Design review of the part built by this model. Coordinates are the model's own, in mm. A direction names the side the tool comes from. Give positions to 0.01 mm unless a question says otherwise; leave off trailing zeros. Write each loop counter-clockwise with the first axis right and the second up, starting at its lowest first coordinate (ties: lowest second). Pieces come first, ordered by that corner, then holes. Notation, with made-up numbers: M 68.25,-10 L 83.25,-10 A19 ccw 83.25,16 Z; hole C -34,37.25 d8. An arc over 180 degrees is marked long. Use a Markdown table: item, result. Add a question column.
Autodesk Inventor part; units mm, degrees
ref_plane "YZ Plane" through (0, 0, 0) normal (1, 0, 0) x (0, 1, 0)
ref_plane "XZ Plane" through (0, 0, 0) normal (0, 1, 0) x (-1, 0, 0)
ref_plane "XY Plane" through (0, 0, 0) normal (0, 0, 1) x (1, 0, 0)
sketch "Sketch1" plane through (0, 0, 0) normal (0, 0, 1) x (1, 0, 0)
  line L0 (-250, -250) -> (250, -250)
  line L1 (250, -250) -> (250, 250)
  line L2 (250, 250) -> (-250, 250)
  line L3 (-250, 250) -> (-250, -250)
  line L4 (-250, -250) -> (250, 250) construction
  line L5 (250, -250) -> (-250, 250) construction
  point P0 (0, 0)
  dimension "d0" = 500
  dimension "d1" = 500
extrude "Extrusion1" add sketch "Sketch1" along normal blind 300
shell "Shell1" thickness 10 removed faces 2 at (83.3333, -83.3333, 0) at (83.3333, -83.3333, 300)
sketch "Sketch2" plane through (0, 0, 0) normal (1, 0, 0) x (0, 1, 0)
  line L0 (-250, 0) -> (250, 0) construction
  line L1 (250, 0) -> (250, 300) construction
  line L2 (-250, 300) -> (250, 300) construction
  line L3 (-250, 0) -> (-250, 300) construction
  line L4 (-250, 0) -> (-250, 300) construction
  line L5 (-250, 150) -> (250, 150) construction
  circle A0 centre (0, 150) radius 30
  arc A1 (205, 115) -> (17.4379, 125.5885) centre (104.6273, 3.5311) ccw
  arc A2 (160.6867, 200) -> (-12.382, 177.3256) centre (111.438, -95.93) ccw
  arc A3 (205, 115) -> (160.6867, 200) centre (150.8369, 140.814) ccw
  point P0 (0, 0)
  dimension "d5" = 60
  dimension "d6" = 300
  dimension "d7" = 150
  dimension "d8" = 60
  dimension "d9" = 35
  dimension "d10" = 205
  dimension "d11" = 50
extrude "Extrusion2" [suppressed]
pattern_linear "Rectangular Pattern1" [suppressed]
pattern_circular "Circular Pattern1" [suppressed]
sketch "Sketch3" plane through (250, -250, 0) normal (1, 0, 0) x (0, 0, -1)
  line L0 (0, 0) -> (0, 500)
  line L1 (0, 500) -> (-300, 500)
  line L2 (-300, 0) -> (-300, 500)
  line L3 (0, 0) -> (-300, 0)
  line L4 (-270, 470) -> (-30, 470)
  line L5 (-30, 470) -> (-30, 30)
  line L6 (-30, 30) -> (-270, 30)
  line L7 (-270, 30) -> (-270, 470)
  point P0 (0, 250)
  dimension "d20" = 30
extrude "Extrusion3" cut sketch "Sketch3" against normal up to surface (10 mm away) contours L4 L5 L6 L7
properties part number "NDM-VOS dummy6"
(1) For pin 1 (3 mm diameter, centred on y = 13, z = 54.5, fed in from +X), flat-tipped, find the tip position at first contact; note if it passes through.
(2) Add section C-C on z = 110.5. Give the boundary of the cut face in (x, y), then the cut area to 3 significant figures.
(3) Machinability: for faces 4 (the flat face through (240, -19, 272)), 5 (the flat face through (-242, 112, 0)), which of the approach directions +Z, -Z, +X, -X, +Y, -Y give a long, thin tool a straight path to every point of the face, cutting with its end or side? Answer none if there is none.
(4) Wall thickness on L1, parallel to Y at x = -203.5, z = 146.5; L2, parallel to X at y = -29, z = 83: over which ranges is each line inside the solid? List them lowest first.
(5) Add section B-B on x = 128. Give the boundary of the cut face in (y, z), then the cut area to 3 significant figures.
(6) Add section A-A on y = -40.5. Give the boundary of the cut face in (x, z), then the cut area to 3 significant figures.
(7) The part is to be moulded in two halves that separate along X. For faces 1 (the flat face through (3, 240, 148)), 2 (the flat face through (-3, -250, 148)), 3 (the flat face through (250, -1, 27)), say which applies: released by +X, released by -X, zero draft, split by the parting line, or undercut.
From the geometry:
| question | item | result |
|---|---|---|
| 1 | pin 1 | stops at x = -240 |
| 2 | outline | M -250,-250 L 250,-250 L 250,-220 L 240,-220 L 240,-240 L -240,-240 L -240,240 L 240,240 L 240,220 L 250,220 L 250,250 L -250,250 Z |
| 2 | area | 15,200 mm^2 |
| 3 | face 4 | +Z, -Z |
| 3 | face 5 | -Z, +X, -X, +Y, -Y |
| 4 | L1 | y = -250 to -240, 240 to 250 |
| 4 | L2 | x = -250 to -240 |
| 5 | outline | M -250,0 L -240,0 L -240,300 L -250,300 Z; M 240,0 L 250,0 L 250,300 L 240,300 Z |
| 5 | area | 6,000 mm^2 |
| 6 | outline | M -250,0 L -240,0 L -240,300 L -250,300 Z; M 240,0 L 250,0 L 250,30 L 240,30 Z; M 240,270 L 250,270 L 250,300 L 240,300 Z |
| 6 | area | 3,600 mm^2 |
| 7 | face 1 | undercut |
| 7 | face 2 | zero draft |
| 7 | face 3 | released by +X |
